CAD build for the part. Positions are in the model's coordinates, mm. Face numbers are marked on the shaded views. A direction names the side the tool comes from. Give positions to 0.01 mm unless a question says otherwise; leave off trailing zeros. Loops run counter-clockwise (first coordinate to the right, second up) from the corner with the lowest first, then second, coordinate; pieces in that order, holes last. Notation, with made-up numbers: M 1,87.25 L 59,87.25 A12 ccw 59,94.25 Z; hole C 81.25,-28 d10. An arc over 180 degrees is marked long. One line per question, with ' | ' between items.
```python
from build123d import *

# Parameters (mm, degrees)
SKETCH1_W                = 100
SKETCH1_H                = 65
BASE_EXTRUDE_DEPTH       = 50
SKETCH2_W                = 35
SKETCH2_H                = 50
CUT_EXTRUDE1_DEPTH       = 130.325171564
SKETCH3_W                = 50
SKETCH3_H                = 31
BOSS_EXTRUDE1_DEPTH      = 50
CUT_EXTRUDE2_DEPTH       = 95.026591983
CHAMFER1_SIZE            = 15
FILLET1_R                = 10
FILLET2_R                = 3
FILLET3_R                = 3
FILLET4_R                = 3
F_8_0_8_DIAMETER_HOLE1_D = 8
F_6_0_6_DIAMETER_HOLE1_D = 6


with BuildPart() as part:
    # Sketch1 → Base-Extrude (new body)
    with BuildSketch(Plane.XY):
        with Locations((0, 32.5)):
            Rectangle(SKETCH1_W, SKETCH1_H)
    extrude(amount=BASE_EXTRUDE_DEPTH)

    # Sketch2 → Cut-Extrude1 (cut, through all)
    with BuildSketch(Plane(origin=(50, 0, 0), x_dir=(0, 0, -1), z_dir=(1, 0, 0))):
        with Locations((-32.5, 40)):
            Rectangle(SKETCH2_W, SKETCH2_H)
    extrude(amount=-CUT_EXTRUDE1_DEPTH, mode=Mode.SUBTRACT)

    # Sketch3 → Boss-Extrude1 (add)
    with BuildSketch(Plane(origin=(0, 15, 0), x_dir=(-1, 0, 0), z_dir=(0, 1, 0))):
        with Locations((0, 30.5)):
            Rectangle(SKETCH3_W, SKETCH3_H)
    extrude(amount=BOSS_EXTRUDE1_DEPTH)

    # Sketch4 → Cut-Extrude2 (cut, through all)
    with BuildSketch(Plane.XY.offset(46)):
        with BuildLine():
            Line((-12, 65), (-12, 40))
            ThreePointArc((-12, 40), (0, 28), (12, 40))
            Line((12, 40), (12, 65))
            Line((12, 65), (-12, 65))
        make_face()
    extrude(amount=-CUT_EXTRUDE2_DEPTH, mode=Mode.SUBTRACT)

    # Chamfer1
    chamfer1_edges = [part.edges().sort_by_distance(p)[0] for p in [
        (18.5, 65, 46),
        (-18.5, 65, 46),
    ]]
    chamfer(chamfer1_edges, length=CHAMFER1_SIZE)

    # Fillet1
    fillet1_edges = [part.edges().sort_by_distance(p)[0] for p in [
        (50, 7.5, 50),
        (-50, 7.5, 50),
        (-50, 65, 7.5),
        (50, 65, 7.5),
    ]]
    fillet(fillet1_edges, radius=FILLET1_R)

    # Fillet2
    fillet2_edges = [part.edges().sort_by_distance(p)[0] for p in [
        (25, 40, 15),
        (-25, 40, 15),
    ]]
    fillet(fillet2_edges, radius=FILLET2_R)

    # Fillet3
    fillet3_edges = [part.edges().sort_by_distance(p)[0] for p in [
        (-25, 32.5, 46),
        (25, 32.5, 46),
    ]]
    fillet(fillet3_edges, radius=FILLET3_R)

    # Fillet4
    fillet4_edges = [part.edges().sort_by_distance(p)[0] for p in [
        (0, 15, 46),
        (25, 15, 30.5),
        (-24.121320344, 15, 45.121320344),
        (24.121320344, 15, 45.121320344),
        (-39, 15, 15),
        (39, 15, 15),
        (-25, 15, 30.5),
        (-25.878679656, 15, 15.878679656),
        (25.878679656, 15, 15.878679656),
    ]]
    fillet(fillet4_edges, radius=FILLET4_R)

    # Ø8.0 (8) Diameter Hole1 (through all)
    with Locations(Plane(origin=(0, 15, 0), x_dir=(1, 0, 0), z_dir=(0, 1, 0))):
        with Locations((40, -40), (-40, -40)):
            Hole(F_8_0_8_DIAMETER_HOLE1_D / 2)

    # Ø6.0 (6) Diameter Hole1 (through all)
    with Locations(Plane(origin=(25, 0, 0), x_dir=(0, 0, -1), z_dir=(1, 0, 0))):
        with Locations((-30, 50)):
            Hole(F_6_0_6_DIAMETER_HOLE1_D / 2)


solid = part.part
```
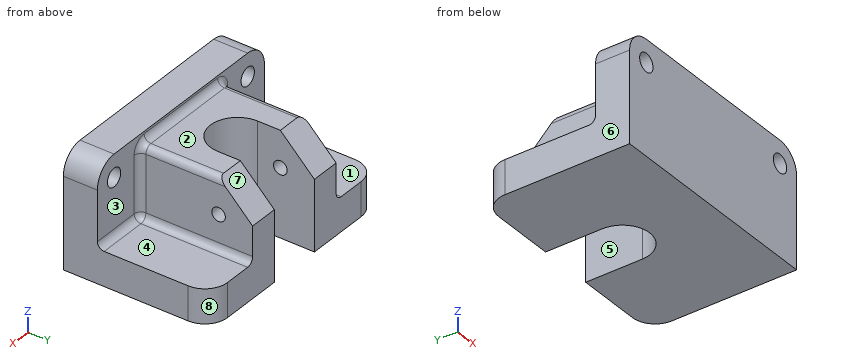
Item 1: Mould opens along X. For the marked faces 5, 6, 7 and 8 say: pulls with the +X half, pulls with the -X half, needs draft (parallel to the pull), parting line crosses it, or undercut.
Conclusion:
face 5: undercut | face 6: pulls with the -X half | face 7: needs draft | face 8: pulls with the +X half
Item 2: Saw through at A-A on x = -15. Give the cut face in (y, z).
Conclusion:
outline: M 0,0 L 65,0 L 65,31 L 50,46 L 18,46 A3 cw 15,49 L 15,50 L 0,50 Z; hole C 50,30 d6
Item 3: Drill centre lines: line 1 along X through (y, z) = (8.5, 40); line 2 along Y through (x, z) = (17.75, 30); line 3 along Z through (x, y) = (40, 10). Where is each one in solid material? Low to high. Write a range as [from, to].
Conclusion:
line 1: [-50, -44], [-36, 36], [44, 50] | line 2: [0, 47], [53, 65] | line 3: [0, 36], [44, 50]
Item 4: Saw through at B-B on z = 24.5. Give the cut face in (x, y).
Conclusion:
outline: M -50,0 L 50,0 L 50,15 L 28,15 A3 cw 25,18 L 25,65 L 12,65 L 12,40 A12 cw -12,40 L -12,65 L -25,65 L -25,18 A3 cw -28,15 L -50,15 Z
Item 5: Saw through at C-C on y = 31.5. Give the cut face in (x, z).
Conclusion:
outline: M -50,0 L -8.47,0 L -8.47,46 L -22,46 A3 ccw -25,43 L -25,18 A3 cw -28,15 L -50,15 Z; M 8.47,0 L 50,0 L 50,15 L 28,15 A3 cw 25,18 L 25,43 A3 ccw 22,46 L 8.47,46 Z
Item 6: Saw through at D-D on x = -31. Give the cut face in (y, z), and give its area (3 significant figures).
Conclusion:
outline: M 0,0 L 65,0 L 65,15 L 18,15 A3 cw 15,18 L 15,50 L 0,50 Z | area: 1,500 mm²
Item 7: Drop flat-ended pins along their axis: P1, Ø5, axis at x = -18, y = 49, coming from the +Z side; P2, Ø5.5, axis at y = 50, z = 30, coming from the +X side; P3, Ø17.5, axis at x = -38.5, y = 36, coming from the +Z side; P4, Ø13, axis at x = 40, z = 40, coming from the +Y side. Give the stop position or say it passes through.
Conclusion:
P1: z = 46 | P2: through | P3: z = 15 | P4: y = 15
Item 8: 3-axis set-ups, long thin cutter, end or side, ignore diameter. For the marked faces 1, 2, 3 and 4: which of +Z, -Z, +X, -X, +Y, -Y reach the whole face in a straight line?
Conclusion:
face 1: +Z, -X, +Y | face 2: +Z, +X, -X, +Y | face 3: +Z, +Y | face 4: +Z, +X, +Y
